Autodesk Inventor part; units mm, degrees
ref_plane "YZ Plane" through (0, 0, 0) normal (1, 0, 0) x (0, 1, 0)
ref_plane "XZ Plane" through (0, 0, 0) normal (0, 1, 0) x (-1, 0, 0)
ref_plane "XY Plane" through (0, 0, 0) normal (0, 0, 1) x (1, 0, 0)
ref_plane "작업 평면1" through (23.5, -8, -2) normal (1, 0, 0) x (0, 0, -1)
sketch "스케치1" plane through (23.5, -8, -2) normal (1, 0, 0) x (0, 0, -1)
  line L0 (0, 16) -> (-8.15, 16)
  line L1 (-8.15, 16) -> (-8.15, 10.6)
  line L2 (-8.15, 10.6) -> (-12.15, 10.6)
  line L3 (-13.15, 9.6) -> (-12.15, 10.6)
  line L4 (-13.15, 9.6) -> (-13.15, 6.4)
  line L5 (-12.15, 5.4) -> (-13.15, 6.4)
  line L6 (-12.15, 5.4) -> (-8.15, 5.4)
  line L7 (-8.15, 5.4) -> (-8.15, 0)
  line L8 (-8.15, 0) -> (0, 0)
  line L9 (0, 16) -> (7.85, 16)
  line L10 (7.85, 16) -> (7.85, 15)
  line L11 (7.85, 15) -> (6.85, 14)
  line L12 (5.85, 14) -> (5.85, 2)
  line L13 (5.85, 14) -> (6.85, 14)
  line L14 (0, 0) -> (7.85, 0)
  line L15 (7.85, 0) -> (7.85, 1)
  line L16 (7.85, 1) -> (6.85, 2)
  line L17 (5.85, 2) -> (6.85, 2)
  line L18 (0, 16) -> (-8.15, 16)
  line L19 (-8.15, 10.6) -> (-12.15, 10.6)
  line L20 (-8.15, 10.6) -> (-12.15, 10.6)
  line L21 (-12.15, 10.6) -> (-13.15, 9.6)
  line L22 (-13.15, 6.4) -> (-12.15, 5.4)
  point P0 (-2, 8)
  dimension "d1" = 7.85
sketch "스케치2" plane through (-23.5, 8, 6.15) normal (0, 0, 1) x (1, 0, 0)
  arc A0 (7.9209, -9.6) -> (7.9209, -6.4) centre (6, -8) ccw
  line L0 (39.0791, -9.6) -> (7.9209, -9.6)
  circle A1 centre (6, -8) radius 2.5
  circle A2 centre (41, -8) radius 2.5
  circle A3 centre (41, -8) radius 2.5
  point P0 (23.5, -8)
  point P1 (7.9209, -6.4)
extrude "돌출1" add sketch "스케치1" against normal up to surface (47 mm away)
extrude "돌출2" cut sketch "스케치2" along normal mid plane 50
sketch "스케치3" plane through (-15.5791, 1.6, 11.15) normal (0, 0, 1) x (1, 0, 0)
  line L0 (15.5791, -14.4593) -> (15.5791, 15.5737)
  line L1 (-7.9209, 4.4) -> (-7.9209, -7.6)
  line L2 (-7.9209, 4.4) -> (11.0791, 4.4)
  line L3 (11.0791, 4.4) -> (11.0791, -7.6)
  line L4 (11.0791, -7.6) -> (-7.9209, -7.6)
  line L5 (-7.9209, -7.6) -> (-7.9209, 4.4)
  line L6 (39.0791, 4.4) -> (39.0791, -7.6)
  line L7 (39.0791, 4.4) -> (20.0791, 4.4)
  line L8 (20.0791, 4.4) -> (20.0791, -7.6)
  line L9 (20.0791, -7.6) -> (39.0791, -7.6)
  line L10 (39.0791, -7.6) -> (39.0791, 4.4)
  point P0 (15.5791, -1.6)
  dimension "d9" = 19
extrude "돌출3" cut sketch "스케치3" against normal up to surface (5 mm away)
properties part number "Bearing Spacer_1.5mmUP"
Input: part model. Units: mm. Frame: model coordinates. A direction names the side the tool comes from. Coordinates: 2 decimals unless noted, no trailing zeros. Write each loop counter-clockwise with the first axis right and the second up, starting at its lowest first coordinate (ties: lowest second). Pieces come first, ordered by that corner, then holes. Notation, with made-up numbers: M 18.25,-14.75 L 65.25,-14.75 A29 cw 65.25,14.25 Z; hole C -26,7 d10. An arc over 180 degrees is marked long. Use one line per item in the form item = value.
Q1. Section A-A (x = 17.5). Return loops of the section in (y, z).
Answer below:
outline = M -8,-9.85 L -7,-9.85 L -6,-8.85 L -6,-7.85 L -2.5,-7.85 L -2.5,6.15 L -8,6.15 Z; M 2.5,-7.85 L 6,-7.85 L 6,-8.85 L 7,-9.85 L 8,-9.85 L 8,6.15 L 2.5,6.15 Z
Q2. Section D-D (z = 4). Return loops of the section in (x, y).
Answer below:
outline = M -23.5,-8 L 23.5,-8 L 23.5,8 L -23.5,8 Z; hole C -17.5,0 d5; hole C 17.5,0 d5
Q3. Section B-B (y = 0). Return loops of the section in (x, z), plus the area to 3 significant figures.
Answer below:
outline = M -23.5,-7.85 L -20,-7.85 L -20,6.15 L -23.5,6.15 Z; M -15,-7.85 L 15,-7.85 L 15,6.15 L 4.5,6.15 L 4.5,11.15 L -4.5,11.15 L -4.5,6.15 L -15,6.15 Z; M 20,-7.85 L 23.5,-7.85 L 23.5,6.15 L 20,6.15 Z
area = 563 mm²
Q4. Material intervals for probe 1 along Y at (x, z) = (-17.5, -3.75); probe 2 along Y at (x, z) = (-5, -8.25); probe 3 along Z at (x, y) = (7, -1), sorted ascending. Write a range as from..to.
Answer below:
probe_1 = -8..-2.5, 2.5..8
probe_2 = -8..-6, 6..8
probe_3 = -7.85..6.15
Q5. Set-up query: faces 1 (the face through (-4.5, 0, 9)), 2 (the face through (4.5, 0, 9)), 3 (the face through (0, 0, -7.85)). Return all of +Z, -Z, +X, -X, +Y, -Y with unobstructed straight access to the full face (end or side cutting, diameter ignored); none if empty.
Answer below:
face_1 = +Z, -X, +Y, -Y
face_2 = +Z, +X, +Y, -Y
face_3 = -Z, +X, -X
Q6. Section C-C (x = -9). Return loops of the section in (y, z).
Answer below:
outline = M -8,-9.85 L -7,-9.85 L -6,-8.85 L -6,-7.85 L 6,-7.85 L 6,-8.85 L 7,-9.85 L 8,-9.85 L 8,6.15 L -8,6.15 Z
Q7. First-contact query: pin 1 (2.5 mm diameter, centred on y = 0, z = 8, fed in from -X); pin 2 (3 mm diameter, centred on x = 1, z = 8.5, fed in from -Y); pin 3 (3 mm diameter, centred on x = 1.5, z = 8, fed in from +Y). Flat tips, straight axial feed; report the tip coordinate or a pass-through.
Answer below:
pin_1 = -4.5
pin_2 = -2.6
pin_3 = 2.6
Q8. Draft query along Y for faces 4 (the face through (0.3, -7.5, -9.85)), 5 (the face through (0, -2.6, 8)), 6 (the face through (0.33, -6.51, -9.36)). Return one class per face: released by +Y, released by -Y, zero draft, split by the parting line, or undercut.
Answer below:
face_4 = zero draft
face_5 = released by -Y
face_6 = undercut
